Verification items for the finished model (mm, model axes). A direction names the side the tool comes from. Round coordinates to 2 decimals unless told otherwise and drop trailing zeros. Write each loop counter-clockwise with the first axis right and the second up, starting at its lowest first coordinate (ties: lowest second). Pieces come first, ordered by that corner, then holes. Notation, with made-up numbers: (14.25, 80) - (25.25, 80) arc R13 ccw to (25.25, 104) - close; hole circle Ø7 at (-29, 18). An arc over 180 degrees is marked (long way). Answer as a JSON object with one key per item and string values.
```python
from build123d import *

# Parameters (mm, degrees)
SKETCH007_W            = 275
SKETCH007_H            = 30
PAD003_DEPTH           = 26
SKETCH008_W            = 9
SKETCH008_H            = 1
POCKET004_DEPTH        = 275
SKETCH009_R            = 1.5
POCKET005_DEPTH        = 6
LINEARPATTERN001_COUNT = 14
LINEARPATTERN001_PITCH = 20
SKETCH017_W            = 29
SKETCH017_H            = 21
SKETCH017_W_2          = 209
POCKET010_DEPTH        = 30
SKETCH018_R            = 1.5
POCKET011_DEPTH        = 275


with BuildPart() as part:
    # Sketch007 → Pad003 (new body)
    with BuildSketch(Plane.XY):
        with Locations((-137.5, 15)):
            Rectangle(SKETCH007_W, SKETCH007_H)
    extrude(amount=PAD003_DEPTH)

    # Sketch008 (on Face2 of Pad003) → Pocket004 (cut)
    with BuildSketch(Plane.YZ):
        with Locations((4.5, 25.5)):
            Rectangle(SKETCH008_W, SKETCH008_H)
    extrude(amount=-POCKET004_DEPTH, mode=Mode.SUBTRACT)

    # Sketch009 (on Face5 of Pocket004) → Pocket005 (cut)
    with BuildSketch(Plane.XY.offset(26)):
        with Locations((-7.5, 4.5)):
            Circle(SKETCH009_R)
    pocket005 = extrude(amount=-POCKET005_DEPTH, mode=Mode.SUBTRACT)

    # LinearPattern001: Pocket005 ×14
    with Locations(*[(-i * LINEARPATTERN001_PITCH, 0, 0) for i in range(1, LINEARPATTERN001_COUNT)]):
        add(pocket005, mode=Mode.SUBTRACT)

    # Sketch017 → Pocket010 (cut)
    with BuildSketch(Plane.XZ):
        with Locations((-14.5, 10.5)):
            Rectangle(SKETCH017_W, SKETCH017_H)
        with Locations((-260.5, 10.5)):
            Rectangle(SKETCH017_W, SKETCH017_H)
        with Locations((-137.5, 10.5)):
            Rectangle(SKETCH017_W_2, SKETCH017_H)
    extrude(amount=-POCKET010_DEPTH, mode=Mode.SUBTRACT)

    # Sketch018 → Pocket011 (cut)
    with BuildSketch(Plane.YZ):
        with Locations((9.4, 18)):
            Circle(SKETCH018_R)
        with Locations((19.4, 18)):
            Circle(SKETCH018_R)
        with Locations((9.4, 3)):
            Circle(SKETCH018_R)
        with Locations((19.4, 3)):
            Circle(SKETCH018_R)
    extrude(amount=-POCKET011_DEPTH, mode=Mode.SUBTRACT)


solid = part.part
```
1. Mould release check, pull along X, two halves, no side actions. Record for faces 6 (the face through (-242, 15, 10)), 7 (the face through (-33, 15, 10)), 8 (the face through (-138, 0, 23)), 9 (the face through (-275, 15, 23)): released by +X, released by -X, zero draft, split by the parting line, or undercut.
Completed:
{"face 6": "undercut", "face 7": "undercut", "face 8": "zero draft", "face 9": "released by -X"}
2. Material ranges on probe 1 along Z at (x, y) = (-31.85, 9.4); probe 2 along X at (y, z) = (8.25, 8.25); probe 3 along Y at (x, z) = (-67.5, 22.6), recorded low to high. Write a range as from..to.
Completed:
{"probe 1": "z = 0..1.5, 4.5..16.5, 19.5..26", "probe 2": "x = -246..-242, -33..-29", "probe 3": "y = 0..3, 6..30"}
3. Access from +Z, -Z, +X, -X, +Y, -Y to the whole of each face (thin tool, end or side, straight path). Record for faces 1 (the face through (-139, 15, 21)), 2 (the face through (-138, 30, 24)), 3 (the face through (-29, 15, 10)), 4 (the face through (-136, 4, 25)), 5 (the face through (-246, 15, 10)).
Completed:
{"face 1": "-Z, +Y, -Y", "face 2": "+Z, -Z, +X, -X, +Y", "face 3": "-Z, +X, +Y, -Y", "face 4": "+Z, +X, -X, -Y", "face 5": "-Z, -X, +Y, -Y"}
4. Go/stop test with flat-tipped pins: pin 1 (4 mm diameter, centred on x = -207.5, y = 4.5, fed in from +Z); pin 2 (5 mm diameter, centred on y = 9.4, z = 3, fed in from +X); pin 3 (8 mm diameter, centred on y = 22, z = 16, fed in from -X); pin 4 (1.8 mm diameter, centred on y = 19.4, z = 3, fed in from -X). Record where each tip stops, or that it passes through.
Completed:
{"pin 1": "stops at z = 25", "pin 2": "stops at x = -29", "pin 3": "stops at x = -246", "pin 4": "passes through"}
5. Cross-section at A-A (x = -42). Record the boundary of the cut face in (y, z), plus the area to 3 significant figures.
Completed:
{"outline": "(0, 21) - (30, 21) - (30, 26) - (9, 26) - (9, 25) - (0, 25) - close", "area": "141 mm^2"}
